```python
from build123d import *

# Parameters (mm, degrees)
BOSS_EXTRUDE1_DEPTH = 104.775
CUT_EXTRUDE1_DEPTH  = 141.290381243
SKETCH2_R           = 2.54
CUT_EXTRUDE2_DEPTH  = 151.322735518


with BuildPart() as part:
    # Model → Boss-Extrude1 (new body)
    with BuildSketch(Plane.XY):
        with BuildLine():
            Line((50.659960212, 72.999871414), (53.774553856, 72.999871414))
            ThreePointArc((53.774553856, 72.999871414), (54.989573754, 72.758188929), (56.019617887, 72.069935444))
            Line((56.019617887, 72.069935444), (59.264200891, 68.825352439))
            ThreePointArc((59.264200891, 68.825352439), (59.477513437, 67.701802895), (58.510322513, 67.091550869))
            Line((58.510322513, 67.091550869), (56.572487817, 67.159221548))
            ThreePointArc((56.572487817, 67.159221548), (55.4691069, 66.130302197), (56.498026251, 65.026921279))
            Line((56.498026251, 65.026921279), (60.677257034, 64.880979325))
            Line((60.677257034, 64.880979325), (62.710657034, 64.880979325))
            ThreePointArc((62.710657034, 64.880979325), (64.129537501, 65.468698857), (64.717257034, 66.887579325))
            Line((64.717257034, 66.887579325), (64.717257034, 68.920979325))
            Line((64.717257034, 68.920979325), (64.57131508, 73.100210108))
            ThreePointArc((64.57131508, 73.100210108), (63.467934162, 74.129129459), (62.439014811, 73.025748542))
            Line((62.439014811, 73.025748542), (62.50668549, 71.087913846))
            ThreePointArc((62.50668549, 71.087913846), (61.896433464, 70.120722922), (60.77288392, 70.334035468))
            Line((60.77288392, 70.334035468), (57.528300915, 73.578618472))
            ThreePointArc((57.528300915, 73.578618472), (56.84004743, 74.608662605), (56.598364945, 75.823682503))
            Line((56.598364945, 75.823682503), (56.598364945, 78.938276147))
            ThreePointArc((56.598364945, 78.938276147), (56.84004743, 80.153296044), (57.528300915, 81.183340177))
            Line((57.528300915, 81.183340177), (60.77288392, 84.427923182))
            ThreePointArc((60.77288392, 84.427923182), (61.896433464, 84.641235728), (62.50668549, 83.674044803))
            Line((62.50668549, 83.674044803), (62.439014811, 81.736210108))
            ThreePointArc((62.439014811, 81.736210108), (63.467934162, 80.63282919), (64.57131508, 81.661748542))
            Line((64.57131508, 81.661748542), (64.717257034, 85.840979325))
            Line((64.717257034, 85.840979325), (64.717257034, 87.874379325))
            ThreePointArc((64.717257034, 87.874379325), (64.129537501, 89.293259792), (62.710657034, 89.880979325))
            Line((62.710657034, 89.880979325), (60.677257034, 89.880979325))
            Line((60.677257034, 89.880979325), (56.498026251, 89.73503737))
            ThreePointArc((56.498026251, 89.73503737), (55.4691069, 88.631656452), (56.572487817, 87.602737101))
            Line((56.572487817, 87.602737101), (58.510322513, 87.67040778))
            ThreePointArc((58.510322513, 87.67040778), (59.477513437, 87.060155754), (59.264200891, 85.93660621))
            Line((59.264200891, 85.93660621), (56.019617887, 82.692023205))
            ThreePointArc((56.019617887, 82.692023205), (54.989573754, 82.00376972), (53.774553856, 81.762087236))
            Line((53.774553856, 81.762087236), (50.659960212, 81.762087236))
            ThreePointArc((50.659960212, 81.762087236), (49.444940315, 82.00376972), (48.414896182, 82.692023205))
            Line((48.414896182, 82.692023205), (45.170313177, 85.93660621))
            ThreePointArc((45.170313177, 85.93660621), (44.957000631, 87.060155754), (45.924191556, 87.67040778))
            Line((45.924191556, 87.67040778), (47.862026251, 87.602737101))
            ThreePointArc((47.862026251, 87.602737101), (48.965407169, 88.631656452), (47.936487817, 89.73503737))
            Line((47.936487817, 89.73503737), (43.757257034, 89.880979325))
            Line((43.757257034, 89.880979325), (41.723857034, 89.880979325))
            ThreePointArc((41.723857034, 89.880979325), (40.304976567, 89.293259792), (39.717257034, 87.874379325))
            Line((39.717257034, 87.874379325), (39.717257034, 85.840979325))
            Line((39.717257034, 85.840979325), (39.863198989, 81.661748542))
            ThreePointArc((39.863198989, 81.661748542), (40.966579907, 80.63282919), (41.995499258, 81.736210108))
            Line((41.995499258, 81.736210108), (41.927828579, 83.674044803))
            ThreePointArc((41.927828579, 83.674044803), (42.538080605, 84.641235728), (43.661630149, 84.427923182))
            Line((43.661630149, 84.427923182), (46.906213154, 81.183340177))
            ThreePointArc((46.906213154, 81.183340177), (47.594466639, 80.153296044), (47.836149123, 78.938276147))
            Line((47.836149123, 78.938276147), (47.836149123, 75.823682503))
            ThreePointArc((47.836149123, 75.823682503), (47.594466639, 74.608662605), (46.906213154, 73.578618472))
            Line((46.906213154, 73.578618472), (43.661630149, 70.334035468))
            ThreePointArc((43.661630149, 70.334035468), (42.538080605, 70.120722922), (41.927828579, 71.087913846))
            Line((41.927828579, 71.087913846), (41.995499258, 73.025748542))
            ThreePointArc((41.995499258, 73.025748542), (40.966579907, 74.129129459), (39.863198989, 73.100210108))
            Line((39.863198989, 73.100210108), (39.717257034, 68.920979325))
            Line((39.717257034, 68.920979325), (39.717257034, 66.887579325))
            ThreePointArc((39.717257034, 66.887579325), (40.304976567, 65.468698857), (41.723857034, 64.880979325))
            Line((41.723857034, 64.880979325), (43.757257034, 64.880979325))
            Line((43.757257034, 64.880979325), (47.936487817, 65.026921279))
            ThreePointArc((47.936487817, 65.026921279), (48.965407169, 66.130302197), (47.862026251, 67.159221548))
            Line((47.862026251, 67.159221548), (45.924191556, 67.091550869))
            ThreePointArc((45.924191556, 67.091550869), (44.957000631, 67.701802895), (45.170313177, 68.825352439))
            Line((45.170313177, 68.825352439), (48.414896182, 72.069935444))
            ThreePointArc((48.414896182, 72.069935444), (49.444940315, 72.758188929), (50.659960212, 72.999871414))
        make_face()
        with BuildLine():
            Line((50.64953831, 75.433607249), (50.269884959, 75.433607249))
            Line((50.269884959, 75.433607249), (50.269884959, 75.8132606))
            ThreePointArc((50.269884959, 75.8132606), (53.985023987, 79.148746278), (50.64953831, 75.433607249))
        make_face(mode=Mode.SUBTRACT)
    extrude(amount=BOSS_EXTRUDE1_DEPTH)

    # Sketch1 → Cut-Extrude1 (cut, through all)
    with BuildSketch(Plane(origin=(64.717257034, 0, 0), x_dir=(0, 0, -1), z_dir=(1, 0, 0))):
        Polygon((-104.775, 89.880979325), (-104.775, 64.880979325), (-61.473729811, 64.880979325), align=None)
    extrude(amount=-CUT_EXTRUDE1_DEPTH, mode=Mode.SUBTRACT)

    # Sketch2 → Cut-Extrude2 (cut, through all)
    with BuildSketch(Plane(origin=(0, 22.041828653, -12.725855706), x_dir=(1, 0, 0), z_dir=(0, -0.8660254037844364, 0.5000000000000041))):
        with Locations(Location((52.217257034, 110.678301344, 0), (0, 0, 232.185356083))):
            Circle(SKETCH2_R)
    extrude(amount=-CUT_EXTRUDE2_DEPTH, mode=Mode.SUBTRACT)


solid = part.part
```
Work out the finished part from the listing and answer in its coordinate system (mm). A direction names the side the tool comes from. Coordinates: 2 decimals unless noted, no trailing zeros.
Q1. Each of these flat-tipped pins is pushed along its axis until it touches: pin 1 Ø3.5 at (x, z) = (52.5, 35.5) entering from +Y; pin 2 Ø8 at (x, z) = (43, 83) entering from -Y; pin 3 Ø0.9 at (x, z) = (52.5, 21) entering from -Y. Where does it stop, or does it pass through?
Q2. Determine the mould class of faces 4 (the face through (52, 81.762, 87)), 5 (the face through (40.32, 89.31, 51.65)), 6 (the face through (40.943, 80.632, 44.699)), 7 (the face through (52, 80.3, 0)) for opening direction X: released by +X, released by -X, zero draft, split by the parting line, or undercut.
Q3. Find the intervals of material crossed by line 1 (Y direction, x = 43, z = 13.5); line 2 (Y direction, x = 56.5, z = 24.5); line 3 (Y direction, x = 47.25, z = 39), in increasing order.
Q4. Which of the six approach directions +Z, -Z, +X, -X, +Y, -Y give full straight-line access (tool end or side, diameter ignored) to faces 1 (the face through (52, 73, 37)), 2 (the face through (52, 81.762, 39)), 3 (the face through (59.47, 87.08, 49.77))?
Findings below:
1. pin 1: stops at y = 81.8
1. pin 2: stops at y = 80.63
1. pin 3: stops at y = 73
2. face 4: undercut
2. face 5: released by -X
2. face 6: undercut
2. face 7: zero draft
3. line 1: y = 64.88 to 70.04, 84.72 to 89.88
3. line 2: y = 65.03 to 67.16, 71.59 to 83.17, 87.6 to 89.74
3. line 3: y = 65 to 67.14, 70.91 to 73.99, 80.78 to 83.86, 87.62 to 89.76
4. face 1: +Z, -Z, -Y
4. face 2: +Z, -Z, +Y
4. face 3: +Z, -Z
